The drawing under review shows one solid part. Ordinate dimensions are in mm from its lowest x, y, z. A direction names the side the tool comes from. Give positions to 0.01 mm unless a question says otherwise; leave off trailing zeros. Order: outer loops, then holes, each group sorted by start corner. A loop starts at its lowest first (then second) coordinate and runs counter-clockwise, first axis right, second up. Notation, with made-up numbers: (-18.75, 58) -> (-9.75, 58) arc R24 ccw to (-9.75, 93) -> close; hole circle Ø6 at (59, -8). An arc over 180 degrees is marked (long way). One line per item, written item: value.
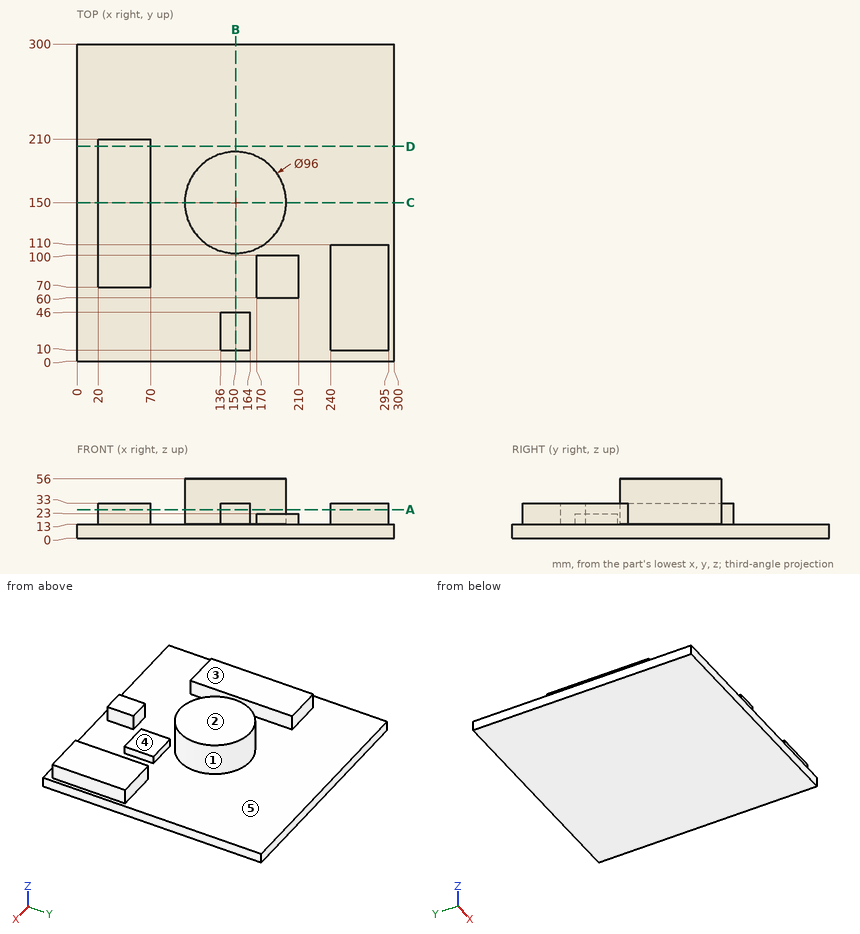
Item 1: To check wall thickness, follow line 1 along X through (y, z) = (45.5, 13.5); line 2 along Y through (x, z) = (147, 31); line 3 along Z through (x, y) = (77.5, 15). State the ranges of each line that lie inside material, in increasing order. Write a range as from..to.
Returned:
line 1: 136..164, 240..295
line 2: 10..46, 102.09..197.91
line 3: 0..13
Item 2: Add section C-C on y = 150. Give the boundary of the cut face in (x, z).
Returned:
outline: (0, 0) -> (300, 0) -> (300, 13) -> (198, 13) -> (198, 56) -> (102, 56) -> (102, 13) -> (70, 13) -> (70, 33) -> (20, 33) -> (20, 13) -> (0, 13) -> close
Item 3: Add section A-A on z = 27. Give the boundary of the cut face in (x, y).
Returned:
outline: (20, 70) -> (70, 70) -> (70, 210) -> (20, 210) -> close; circle Ø96 at (150, 150); (136, 10) -> (164, 10) -> (164, 46) -> (136, 46) -> close; (240, 10) -> (295, 10) -> (295, 110) -> (240, 110) -> close
Item 4: Add section D-D on y = 203. Give the boundary of the cut face in (x, z).
Returned:
outline: (0, 0) -> (300, 0) -> (300, 13) -> (70, 13) -> (70, 33) -> (20, 33) -> (20, 13) -> (0, 13) -> close
Item 5: Machinability: for the marked faces 1 and 2, which of the approach directions +Z, -Z, +X, -X, +Y, -Y give a long, thin tool a straight path to every point of the face, cutting with its end or side? Answer none if there is none.
Returned:
face 1: +Z
face 2: +Z, +X, -X, +Y, -Y
Item 6: Draft analysis for pull direction X (two halves, no side actions). For the marked faces 3, 4 and 5, state which applies: pulls with the +X half, pulls with the -X half, needs draft (parallel to the pull), parting line crosses it, or undercut.
Returned:
face 3: needs draft
face 4: undercut
face 5: undercut
Item 7: Add section B-B on x = 150. Give the boundary of the cut face in (y, z).
Returned:
outline: (0, 0) -> (300, 0) -> (300, 13) -> (198, 13) -> (198, 56) -> (102, 56) -> (102, 13) -> (46, 13) -> (46, 33) -> (10, 33) -> (10, 13) -> (0, 13) -> close
Item 8: Clearance check with flat-ended pins moving along their axes: P1, Ø6, axis at y = 84, z = 26.5, coming from the +X side; P2, Ø11, axis at y = 82, z = 15.5, coming from the +X side; P3, Ø20, axis at x = 198, y = 85, coming from the +Z side; P4, Ø15, axis at x = 55.5, y = 124, coming from the +Z side. State where each tip first meets the part, or that it passes through.
Returned:
P1: x = 295
P2: x = 300
P3: z = 23
P4: z = 33
